Read the model definition and answer for the solid it produces. Units are mm, in the model's axes. Face numbers are marked on the shaded views. A direction names the side the tool comes from. Round coordinates to 2 decimals unless told otherwise and drop trailing zeros. Loops run counter-clockwise (first coordinate to the right, second up) from the corner with the lowest first, then second, coordinate; pieces in that order, holes last. Notation, with made-up numbers: (69, -30.75) -> (95, -30.75) arc R10 ccw to (95, -17.75) -> close; hole circle Ø1 at (-3, -21.75). An arc over 180 degrees is marked (long way). Put each result on its own line as item: value.
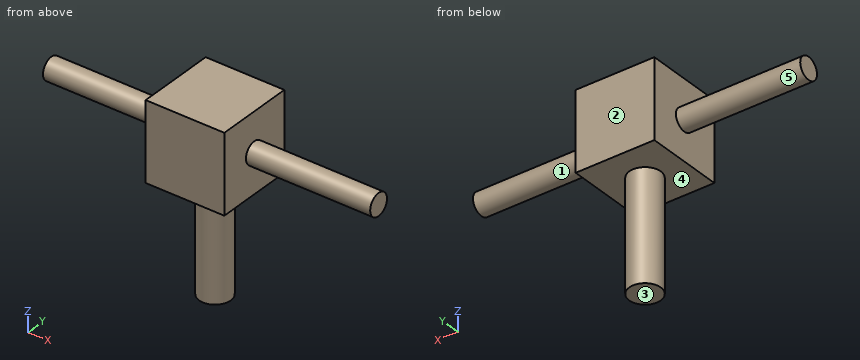
from build123d import *

# Parameters (mm, degrees)
F0_W          = 31.75
F0_H          = 31.75
F1_DEPTH      = 15.875
F2_R          = 4.445
F3_DEPTH      = 50.165
F3_DEPTH_BACK = 81.915
F4_R          = 6.35
F5_DEPTH      = 44.45


with BuildPart() as f1:
    # F0 (on Front) → F1 (new body, symmetric)
    with BuildSketch(Plane.XZ):
        with Locations((-15.875, 15.875)):
            Rectangle(F0_W, F0_H)
    extrude(amount=F1_DEPTH, both=True)

    # F2 (on face) → F3 (join, two sides)
    with BuildSketch(Plane.YZ) as f3_sk:
        with Locations((0, 15.875)):
            Circle(F2_R)
    extrude(amount=F3_DEPTH)
    extrude(f3_sk.sketch, amount=-F3_DEPTH_BACK)

    # F4 (on face) → F5 (join)
    with BuildSketch(Plane(origin=(0, 0, 0), x_dir=(1, 0, 0), z_dir=(0, 0, -1))):
        with Locations((-15.875, 0)):
            Circle(F4_R)
    extrude(amount=F5_DEPTH)


solid = f1.part
Item 1: The part is cut by section A-A (y = 0). Determine the outline of the cut face in (x, z) (3 decimals).
Derived:
outline: (-81.915, 11.43) -> (-31.75, 11.43) -> (-31.75, 0) -> (-22.225, 0) -> (-22.225, -44.45) -> (-9.525, -44.45) -> (-9.525, 0) -> (0, 0) -> (0, 11.43) -> (50.165, 11.43) -> (50.165, 20.32) -> (0, 20.32) -> (0, 31.75) -> (-31.75, 31.75) -> (-31.75, 20.32) -> (-81.915, 20.32) -> close
Item 2: The part is cut by section C-C (x = 24). Determine the outline of the cut face in (y, z) (3 decimals).
Derived:
outline: circle Ø8.89 at (0, 15.875)
Item 3: Flat-ended cylindrical pins translate along their axes: pin 1 Ø4 at (x, z) = (3, 22.5) entering from +Y; pin 2 Ø3 at (y, z) = (-9, 20.5) entering from +X; pin 3 Ø6 at (y, z) = (-7, -30) entering from -X. Find the tip coordinate at first contact, or state that the pin passes through.
Derived:
pin 1: passes through
pin 2: stops at x = 0
pin 3: stops at x = -20.81
Item 4: Which of the six approach directions +Z, -Z, +X, -X, +Y, -Y give full straight-line access (tool end or side, diameter ignored) to the marked faces 1, 2, 3, 4 and 5?
Derived:
face 1: +X
face 2: +Z, -Z, +X, -X, +Y
face 3: -Z, +X, -X, +Y, -Y
face 4: -Z
face 5: -X
Item 5: Find the intervals of material crossed by line 1 along Z through (x, y) = (-13, 10.5); line 2 along X through (y, z) = (-13, 12.5); line 3 along Y through (x, z) = (25.5, 18), in increasing order.
Derived:
line 1: z = 0 to 31.75
line 2: x = -31.75 to 0
line 3: y = -3.9 to 3.9
Item 6: The part is cut by section D-D (z = -5). Determine the outline of the cut face in (x, y) (3 decimals), then the cut area to 3 significant figures.
Derived:
outline: circle Ø12.7 at (-15.875, 0)
area: 127 mm^2
Item 7: The part is cut by section B-B (z = 26). Determine the outline of the cut face in (x, y) (3 decimals), then the cut area to 3 significant figures.
Derived:
outline: (-31.75, -15.875) -> (0, -15.875) -> (0, 15.875) -> (-31.75, 15.875) -> close
area: 1,010 mm^2
